Design review of the part built by this model. Coordinates are the model's own, in mm. A direction names the side the tool comes from. Coordinates: 2 decimals unless noted, no trailing zeros. Write each loop counter-clockwise with the first axis right and the second up, starting at its lowest first coordinate (ties: lowest second). Pieces come first, ordered by that corner, then holes. Notation, with made-up numbers: M 59,70.25 L 108,70.25 A21 cw 108,82.25 Z; hole C 10,11.5 d5. An arc over 180 degrees is marked long. Write item = value, one per line.
```python
from build123d import *

# Parameters (mm, degrees)
SKETCH1_R                   = 1.6
BASE_FLANGE1_DEPTH          = 0.4
SKETCHED_START              = 45.702497433
SKETCHED_BEND8_DEPTH        = 12
SKETCHED_BEND8_2_DEPTH      = 8
SKETCHED_START_2            = 53.702497433
SKETCHED_BEND8_3_DEPTH      = 4
SKETCHED_START_3            = -0.4
SKETCHED_BEND12_OUTLINE_W   = 12
SKETCHED_BEND12_OUTLINE_H   = 0.4
SKETCHED_BEND12_DEPTH       = 14.907300918
SKETCHED_START_4            = 0.242920367
SKETCHED_BEND12_2_OUTLINE_W = 0.4
SKETCHED_BEND12_2_OUTLINE_H = 4.8
SKETCHED_BEND12_2_DEPTH     = 12
SKETCHED_START_5            = 12.485840735
SKETCHED_BEND12_3_DEPTH     = 0.4
SKETCHED_BEND12_4_OUTLINE_W = 9
SKETCHED_BEND12_4_OUTLINE_H = 0.4
SKETCHED_BEND12_4_DEPTH     = 8
SKETCHED_START_6            = 3.742920367
SKETCHED_BEND12_5_OUTLINE_W = 0.4
SKETCHED_BEND12_5_OUTLINE_H = 3.2
SKETCHED_BEND12_5_DEPTH     = 5
SKETCHED_BEND12_6_OUTLINE_W = 0.4
SKETCHED_BEND12_6_OUTLINE_H = 20
SKETCHED_BEND12_6_DEPTH     = 12.485840735
SKETCHED_START_7            = -4.042672779
SKETCHED_BEND12_7_DEPTH     = 33.307300919
SKETCHED_START_8            = 8.957327221
SKETCHED_BEND12_8_DEPTH     = 20
FILLET1_R                   = 3
FILLET2_R                   = 1
FILLET3_R                   = 1


with BuildPart() as part:
    # Base-Flange1: sheet metal written as solids
    # Sketch1 → Base-Flange1 (new body)
    with BuildSketch(Plane.XY):
        Polygon((30.702497433, -1.042672779), (30.702497433, 8.957327221), (45.702497433, 8.957327221), (45.702497433, 3.957327221), (49.202497433, 3.957327221), (49.202497433, 0.757327221), (45.702497433, 0.757327221), (45.702497433, -4.042672779), (57.702497433, -4.042672779), (57.702497433, 0.757327221), (54.202497433, 0.757327221), (54.202497433, 3.957327221), (57.702497433, 3.957327221), (57.702497433, 8.957327221), (72.702497433, 8.957327221), (72.702497433, 26.957327221), (63.702497433, 26.957327221), (63.702497433, 28.957327221), (57.702497433, 28.957327221), (57.702497433, 34.957327221), (53.702497433, 34.957327221), (53.702497433, 43.957327221), (45.702497433, 43.957327221), (45.702497433, 28.957327221), (20.702497433, 28.957327221), (20.702497433, -1.042672779), align=None)
        with Locations((25.702497433, 3.957327221)):
            Circle(SKETCH1_R, mode=Mode.SUBTRACT)
    extrude(amount=-BASE_FLANGE1_DEPTH)

    # Sketched Bend8: read off the stored shape, not the designer's step
    # Sketched Bend8 outline → Sketched Bend8 (cut)
    with BuildSketch(Plane.YZ.offset(SKETCHED_START)):
        with BuildLine():
            ThreePointArc((29.597083672, 0), (29.338793878, -0.291607978), (28.96462814, -0.4))
            Line((28.96462814, -0.4), (43.957327221, -0.4))
            Line((43.957327221, -0.4), (43.957327221, 0))
            Line((43.957327221, 0), (29.597083672, 0))
        make_face()
    extrude(amount=SKETCHED_BEND8_DEPTH, mode=Mode.SUBTRACT)

    # Sketched Bend8 2 outline → Sketched Bend8 2 (add)
    with BuildSketch(Plane.YZ.offset(SKETCHED_START)):
        with BuildLine():
            Line((29.66462814, 14.507300918), (29.26462814, 14.507300918))
            Line((29.26462814, 14.507300918), (29.26462814, 0.3))
            ThreePointArc((29.26462814, 0.3), (29.176760174, 0.087867966), (28.96462814, 0))
            Line((28.96462814, 0), (29.597083672, 0))
            ThreePointArc((29.597083672, 0), (29.647533284, 0.146245118), (29.66462814, 0.3))
            Line((29.66462814, 0.3), (29.66462814, 14.507300918))
        make_face()
    extrude(amount=SKETCHED_BEND8_2_DEPTH)

    # Sketched Bend8 3 outline → Sketched Bend8 3 (add)
    with BuildSketch(Plane.YZ.offset(SKETCHED_START_2)):
        with BuildLine():
            Line((29.66462814, 0.3), (29.66462814, 5.507300918))
            Line((29.66462814, 5.507300918), (29.26462814, 5.507300918))
            Line((29.26462814, 5.507300918), (29.26462814, 0.3))
            ThreePointArc((29.26462814, 0.3), (29.176760174, 0.087867966), (28.96462814, 0))
            Line((28.96462814, 0), (29.597083672, 0))
            ThreePointArc((29.597083672, 0), (29.647533284, 0.146245118), (29.66462814, 0.3))
        make_face()
    extrude(amount=SKETCHED_BEND8_3_DEPTH)

    # Sketched Bend12: read off the stored shape, not the designer's step
    # Sketched Bend12 outline → Sketched Bend12 (cut)
    with BuildSketch(Plane.XY.offset(SKETCHED_START_3)):
        with Locations((51.702497433, 29.46462814)):
            Rectangle(SKETCHED_BEND12_OUTLINE_W, SKETCHED_BEND12_OUTLINE_H)
    extrude(amount=SKETCHED_BEND12_DEPTH, mode=Mode.SUBTRACT)



with BuildPart() as body_2:
    # Sketched Bend12 2 outline → Sketched Bend12 2 (new body)
    with BuildSketch(Plane.XY.offset(SKETCHED_START_4)):
        with BuildLine():
            ThreePointArc((45.545417801, 28.96462814), (45.340392547, 29.459602886), (44.845417801, 29.66462814))
            Line((44.845417801, 29.66462814), (39.638116882, 29.66462814))
            Line((39.638116882, 29.66462814), (39.638116882, 29.26462814))
            Line((39.638116882, 29.26462814), (44.845417801, 29.26462814))
            ThreePointArc((44.845417801, 29.26462814), (45.057549835, 29.176760174), (45.145417801, 28.96462814))
            Line((45.145417801, 28.96462814), (45.145417801, 3.957327221))
            Line((45.145417801, 3.957327221), (45.545417801, 3.957327221))
            Line((45.545417801, 3.957327221), (45.545417801, 28.96462814))
        make_face()
        with Locations((45.345417801, -1.642672779)):
            Rectangle(SKETCHED_BEND12_2_OUTLINE_W, SKETCHED_BEND12_2_OUTLINE_H)
    extrude(amount=SKETCHED_BEND12_2_DEPTH)

    # Sketched Bend12 4 outline → Sketched Bend12 4 (add)
    with BuildSketch(Plane.XY.offset(SKETCHED_START_4)):
        with Locations((35.138116882, 29.46462814)):
            Rectangle(SKETCHED_BEND12_4_OUTLINE_W, SKETCHED_BEND12_4_OUTLINE_H)
    extrude(amount=SKETCHED_BEND12_4_DEPTH)

    # Sketched Bend12 5 outline → Sketched Bend12 5 (add)
    with BuildSketch(Plane.XY.offset(SKETCHED_START_6)):
        with Locations((45.345417801, 2.357327221)):
            Rectangle(SKETCHED_BEND12_5_OUTLINE_W, SKETCHED_BEND12_5_OUTLINE_H)
    extrude(amount=SKETCHED_BEND12_5_DEPTH)


with BuildPart() as body_3:
    # Sketched Bend12 3 outline → Sketched Bend12 3 (new body)
    with BuildSketch(Plane.XY.offset(SKETCHED_START_5)):
        Polygon((45.145417801, 8.957327221), (45.145417801, 28.957327221), (39.702497433, 28.957327221), (39.702497433, 26.957327221), (30.702497433, 26.957327221), (30.702497433, 8.957327221), align=None)
    extrude(amount=SKETCHED_BEND12_3_DEPTH)


with BuildPart() as part_1:
    add(part.part)

    add(body_2.part)  # Sketched Bend12 6 merges body 2

    add(body_3.part)  # Sketched Bend12 6 merges body 3
    # Sketched Bend12 6 outline → Sketched Bend12 6 (add)
    with BuildSketch(Plane.XY):
        with Locations((45.345417801, 18.957327221)):
            Rectangle(SKETCHED_BEND12_6_OUTLINE_W, SKETCHED_BEND12_6_OUTLINE_H)
    extrude(amount=SKETCHED_BEND12_6_DEPTH)

    # Sketched Bend12 7 outline → Sketched Bend12 7 (cut)
    with BuildSketch(Plane(origin=(0, 0, 0), x_dir=(1, 0, 0), z_dir=(0, 1, 0)).offset(SKETCHED_START_7)):
        with BuildLine():
            ThreePointArc((45.145417801, 0.4), (45.428260513, 0.282842712), (45.545417801, 0))
            Line((45.545417801, 0), (45.702497433, 0))
            Line((45.702497433, 0), (45.702497433, -14))
            Line((45.702497433, -14), (57.702497433, -14))
            Line((57.702497433, -14), (57.702497433, 0))
            Line((57.702497433, 0), (72.702497433, 0))
            Line((72.702497433, 0), (72.702497433, 0.4))
            Line((72.702497433, 0.4), (45.145417801, 0.4))
        make_face()
    extrude(amount=SKETCHED_BEND12_7_DEPTH, mode=Mode.SUBTRACT)

    # Sketched Bend12 8 outline → Sketched Bend12 8 (add)
    with BuildSketch(Plane(origin=(0, 0, 0), x_dir=(1, 0, 0), z_dir=(0, 1, 0)).offset(SKETCHED_START_8)):
        with BuildLine():
            Line((45.145417801, -12.485840735), (45.145417801, -12.885840735))
            ThreePointArc((45.145417801, -12.885840735), (45.428260513, -12.768683447), (45.545417801, -12.485840735))
            Line((45.545417801, -12.485840735), (45.145417801, -12.485840735))
        make_face()
    extrude(amount=SKETCHED_BEND12_8_DEPTH)

    # Fillet1
    fillet1_edges = [part_1.edges().sort_by_distance(p)[0] for p in [
        (45.345417801, -4.042672779, 0.242920367),
        (45.345417801, -4.042672779, 12.242920367),
        (30.702497433, -1.042672779, -0.2),
        (20.702497433, -1.042672779, -0.2),
    ]]
    fillet(fillet1_edges, radius=FILLET1_R)

    # Fillet2
    fillet2_edges = [part_1.edges().sort_by_distance(p)[0] for p in [
        (20.702497433, 28.957327221, -0.2),
        (30.702497433, 26.957327221, 12.685840735),
        (30.702497433, 8.957327221, 12.685840735),
        (30.638116882, 29.46462814, 0.242920367),
        (30.638116882, 29.46462814, 8.242920367),
    ]]
    fillet(fillet2_edges, radius=FILLET2_R)

    # Fillet3
    fillet3_edges = [part_1.edges().sort_by_distance(p)[0] for p in [
        (45.345417801, 3.957327221, 0.242920367),
        (45.345417801, 3.957327221, 3.742920367),
        (45.345417801, 0.757327221, 3.742920367),
        (45.345417801, 0.757327221, 0.242920367),
        (45.345417801, 0.757327221, 12.242920367),
        (45.345417801, 0.757327221, 8.742920367),
        (45.345417801, 3.957327221, 8.742920367),
        (45.345417801, 3.957327221, 12.242920367),
    ]]
    fillet(fillet3_edges, radius=FILLET3_R)


solid = part_1.part
```
Q1. Consider section C-C, the plane y = 3.5. State the section outline as (x, z) points.
Check result:
outline = M 20.7,-0.4 L 24.17,-0.4 L 24.17,0 L 20.7,0 Z; M 27.24,-0.4 L 30.7,-0.4 L 30.7,0 L 27.24,0 Z; M 45.15,3.58 L 45.55,3.58 L 45.55,8.9 L 45.15,8.9 Z
Q2. Consider section A-A, the plane x = 43.5. State the section outline as (y, z) points.
Check result:
outline = M 8.96,-0.4 L 28.96,-0.4 L 28.96,0 L 8.96,0 Z; M 8.96,12.49 L 28.96,12.49 L 28.96,12.89 L 8.96,12.89 Z; M 29.26,0.24 L 29.66,0.24 L 29.66,12.24 L 29.26,12.24 Z
Q3. For P1, Ø4, axis at y = 1, z = 10.5, coming from the -X side; P2, Ø0.5, axis at x = 41, z = 12.5, coming from the -Y side; P3, Ø0.8, axis at x = 42, y = 29, coming from the -Z side, all flat-tipped, find the tip position at first contact; note any pin that passes through.
Check result:
P1 = 45.15
P2 = 8.96
P3 = -0.4
Q4. The part is to be moulded in two halves that separate along Y. For faces 1 (the cylindrical face through (30.939, 29.467, 0.528)), 2 (the cylindrical face through (30.99, 26.66, 12.69)), 3 (the cylindrical face through (45.35, -3.14, 1.1)), 4 (the cylindrical face through (45.35, 4.24, 11.94)), say which applies: +Y half, -Y half, draft (parallel to the pull), parting line (faces both ways), or undercut.
Check result:
face_1 = draft
face_2 = +Y half
face_3 = -Y half
face_4 = undercut
Q5. Machinability: for faces 5 (the cylindrical face through (31.003, 9.242, 12.689)), 6 (the cylindrical face through (45.348, 1.042, 9.044)), 7 (the flat face through (33, 18, 0)), 8 (the cylindrical face through (45.348, 3.657, 3.458)), 9 (the flat face through (38, 19, 12.886)), which of the approach directions +Z, -Z, +X, -X, +Y, -Y give a long, thin tool a straight path to every point of the face, cutting with its end or side? Answer none if there is none.
Check result:
face_5 = +Z, -X, -Y
face_6 = +Z, +X, -X
face_7 = -X, +Y, -Y
face_8 = -Z, +X, -X
face_9 = +Z, +X, -X, +Y, -Y
Q6. Consider section B-B, the plane z = 10.5. State the section outline as (x, y) points, and give its area (3 significant figures).
Check result:
outline = M 39.64,29.26 L 44.85,29.26 A0.3 cw 45.15,28.96 L 45.15,3.96 L 45.55,3.96 L 45.55,28.96 A0.7 ccw 44.85,29.66 L 39.64,29.66 Z; M 45.15,-3.77 L 45.55,-3.77 L 45.55,0.76 L 45.15,0.76 Z
area = 14.2 mm²
Q7. Wall thickness on line 1 (Z direction, x = 39.75, y = 17.5); line 2 (X direction, y = 12, z = 0.5); line 3 (Y direction, x = 33.5, z = 3): over which ranges is each line inside the solid? List them lowest first.
Check result:
line_1 = -0.4 to 0, 12.49 to 12.89
line_2 = 45.15 to 45.55
line_3 = 29.26 to 29.66
Q8. Consider section D-D, the plane x = 26. State the section outline as (y, z) points.
Check result:
outline = M -1.04,-0.4 L 2.39,-0.4 L 2.39,0 L -1.04,0 Z; M 5.53,-0.4 L 28.96,-0.4 L 28.96,0 L 5.53,0 Z
